For this review, take the finished solid that the model builds, in its own axes (mm). Round coordinates to 2 decimals unless told otherwise and drop trailing zeros. Order: outer loops, then holes, each group sorted by start corner. A loop starts at its lowest first (then second) coordinate and runs counter-clockwise, first axis right, second up. Notation, with made-up numbers: (48, 80) -> (92, 80) arc R24 ccw to (92, 109) -> close; hole circle Ø10 at (-2, 53). An arc over 180 degrees is marked (long way). Use a Markdown table: item, result. Add a question column.
1) Wall thickness on line 1 along Z through (x, y) = (434.5, 50.5) (3 decimals); line 2 along Y through (x, z) = (222, -50); line 3 along Y through (x, z) = (443, -44.5): over which ranges is each line inside the solid? List them lowest first. Write a range as [from, to].
2) Consider section A-A (x = 246.5). State the section outline as (y, z) points.
3) Clearance check with a flat-ended pin moving along its axis: P1, Ø1, axis at y = 51, z = -72.5, coming from the +X side. State where the tip first meets the part, or that it passes through.
4) Consider section B-B (y = 50). State the section outline as (x, z) points.
5) Consider section C-C (z = -50). State the section outline as (x, y) points.
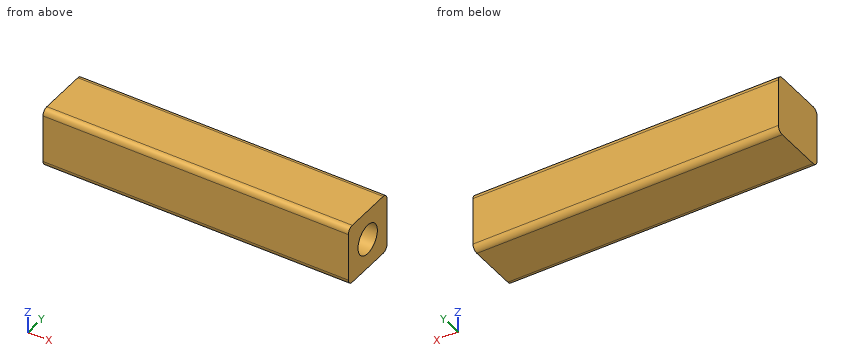
Autodesk Inventor part; units mm, degrees
ref_plane "YZ Plane" through (0, 0, 0) normal (1, 0, 0) x (0, 1, 0)
ref_plane "XZ Plane" through (0, 0, 0) normal (0, 1, 0) x (-1, 0, 0)
ref_plane "XY Plane" through (0, 0, 0) normal (0, 0, 1) x (1, 0, 0)
sketch "Sketch1" plane through (0, 0, 0) normal (1, 0, 0) x (0, 1, 0)
  line L0 (0, 0) -> (100, 0)
  line L1 (100, 0) -> (100, -100)
  line L2 (100, -100) -> (0, -100)
  line L3 (0, -100) -> (0, 0)
  circle A0 centre (50, -50) radius 25
  line L4 (50, 0) -> (50, -50)
  line L5 (50, -50) -> (0, -50)
  dimension "d0" = 100
  dimension "d1" = 100
  dimension "d4" = 50
  dimension "d8" = 50
  dimension "d9" = 50
extrude "Extrusion1" add sketch "Sketch1" along normal blind 500 contours L0 L4 A0 L5 L3 | L0 L1 L2 L3 L5 A0 L4
extrude "Extrusion2" add sketch "Sketch1" against normal blind 10
fillet "Fillet1" radius 10 4 edges at (245, 100, 0) (245, 0, 0) (245, 0, -100) (245, 100, -100)
properties part number "Contenedor"
Results list:
| question | item | result |
|---|---|---|
| 1 | line 1 | [-100, -74.995], [-25.005, 0] |
| 1 | line 2 | [0, 25], [75, 100] |
| 1 | line 3 | [0, 25.61], [74.39, 100] |
| 2 | outline | (0, -90) arc R10 ccw to (10, -100) -> (90, -100) arc R10 ccw to (100, -90) -> (100, -10) arc R10 ccw to (90, 0) -> (10, 0) arc R10 ccw to (0, -10) -> close; hole circle Ø50 at (50, -50) |
| 3 | P1 | x = 0 |
| 4 | outline | (-10, -100) -> (500, -100) -> (500, -75) -> (0, -75) -> (0, -25) -> (500, -25) -> (500, 0) -> (-10, 0) -> close |
| 5 | outline | (-10, 0) -> (500, 0) -> (500, 25) -> (0, 25) -> (0, 75) -> (500, 75) -> (500, 100) -> (-10, 100) -> close |
